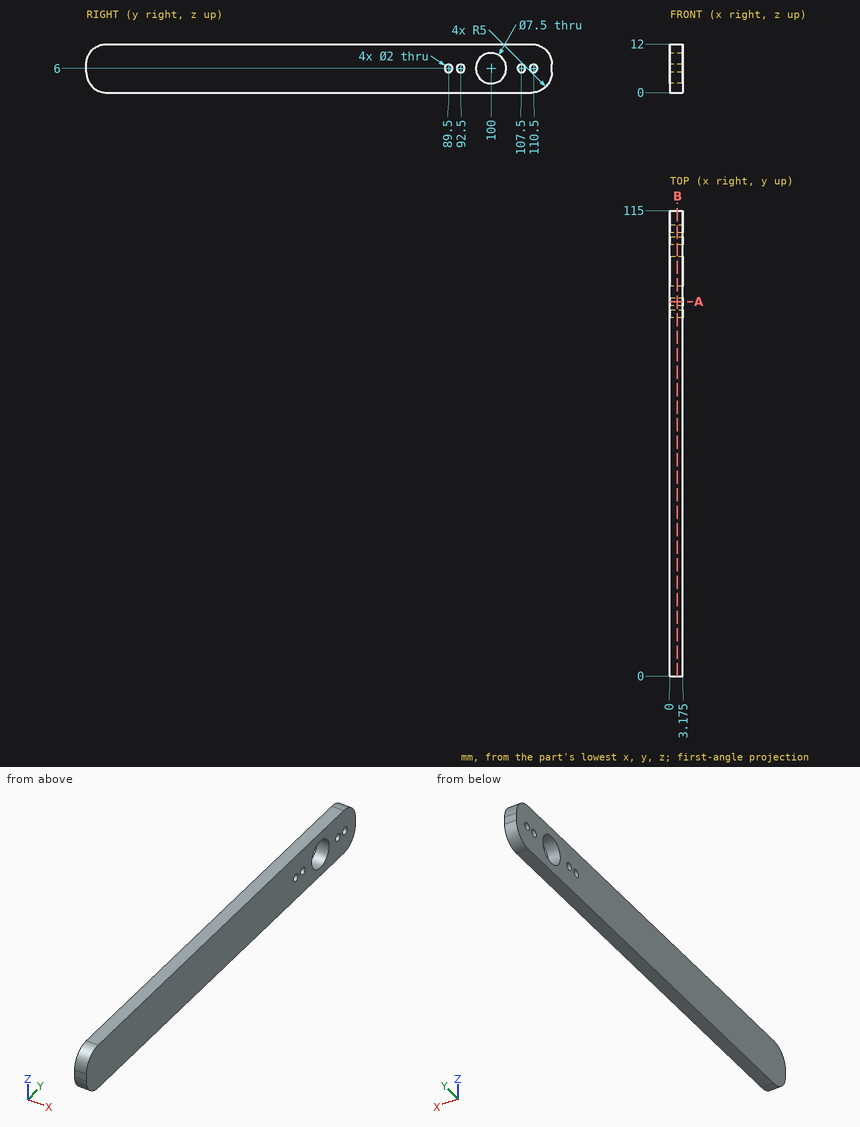
Can you work these out from the drawing? Everything is in mm from the part's minimum corner. Give positions to 0.01 mm unless a question says otherwise; leave off trailing zeros. Order: outer loops, then holes, each group sorted by start corner. A loop starts at its lowest first (then second) coordinate and runs counter-clockwise, first axis right, second up. Notation, with made-up numbers: (8.5, -37.5) -> (34.5, -37.5) arc R12 ccw to (34.5, -27.5) -> close; hole circle Ø11 at (-32, -9.75). An arc over 180 degrees is marked (long way). Return JSON: item names as keys, results as strings.
1. For pin 1 Ø1.8 at (y, z) = (107.5, 6) entering from +X; pin 2 Ø2.5 at (y, z) = (92.5, 6) entering from +X (3 decimals), each with a flat end and sliding along its axis, tell me the tip position at first contact or that it passes through.
Answer list:
{"pin 1": "passes through", "pin 2": "stops at x = 3.175"}
2. Imagine slicing it at A-A on y = 92.5. List the corners of the cut face in (x, z) for me (3 decimals), then the cut area to 4 significant figures.
Answer list:
{"outline": "(0, 0) -> (3.175, 0) -> (3.175, 5) -> (0, 5) -> close; (0, 7) -> (3.175, 7) -> (3.175, 12) -> (0, 12) -> close", "area": "31.75 mm2"}
3. Imagine slicing it at B-B on x = 1.9. List the corners of the cut face in (y, z) for me, then the cut area to 3 significant figures.
Answer list:
{"outline": "(0, 5) arc R5 ccw to (5, 0) -> (110, 0) arc R5 ccw to (115, 5) -> (115, 7) arc R5 ccw to (110, 12) -> (5, 12) arc R5 ccw to (0, 7) -> close; hole circle Ø2 at (89.5, 6); hole circle Ø2 at (92.5, 6); hole circle Ø7.5 at (100, 6); hole circle Ø2 at (107.5, 6); hole circle Ø2 at (110.5, 6)", "area": "1,300 mm2"}
4. I need wall thicknesses on line 1 (Z direction, x = 2, y = 89.5); line 2 (Z direction, x = 1.45, y = 100); line 3 (Y direction, x = 1.55, z = 3). Which ranges of each line are inside material? Lowest first, please. Write a range as from..to.
Answer list:
{"line 1": "z = 0..5, 7..12", "line 2": "z = 0..2.25, 9.75..12", "line 3": "y = 0.42..97.75, 102.25..114.58"}
